For this review, take the finished solid that the model builds, in its own axes (mm). A direction names the side the tool comes from. Round coordinates to 2 decimals unless told otherwise and drop trailing zeros. Write each loop counter-clockwise with the first axis right and the second up, starting at its lowest first coordinate (ties: lowest second). Pieces come first, ordered by that corner, then holes.
from build123d import *

# Parameters (mm, degrees)
SKETCH1_R           = 11.7729
SKETCH1_R_2         = 1.016
BOSS_EXTRUDE1_DEPTH = 1.6256
SKETCH2_R           = 0.762
CUT_EXTRUDE1_DEPTH  = 17.728566112
SKETCH3_R           = 3.3655
SKETCH3_R_2         = 2.2606
BOSS_EXTRUDE2_DEPTH = 2.54
SKETCH4_R           = 2.6924
BOSS_EXTRUDE3_DEPTH = 0.8636
SKETCH5_R           = 2.2606
CUT_EXTRUDE2_DEPTH  = 1.27


with BuildPart() as part:
    # Sketch1 → Boss-Extrude1 (new body)
    with BuildSketch(Plane(origin=(0, 0, 0), x_dir=(1, 0, 0), z_dir=(0, 1, 0))):
        with Locations(Location((0, 0, 0), (0, 0, 270))):
            Circle(SKETCH1_R)
        with Locations(Location((0, 0, 0), (0, 0, 270))):
            Circle(SKETCH1_R_2, mode=Mode.SUBTRACT)
    extrude(amount=BOSS_EXTRUDE1_DEPTH)

    # Sketch2 → Cut-Extrude1 (cut, through all)
    with BuildSketch(Plane(origin=(0, 1.6256, 0), x_dir=(1, 0, 0), z_dir=(0, 1, 0))):
        with Locations(Location((8.0518, 0, 0), (0, 0, 270))):
            Circle(SKETCH2_R)
        with Locations(Location((-8.0518, 0, 0), (0, 0, 270))):
            Circle(SKETCH2_R)
    extrude(amount=-CUT_EXTRUDE1_DEPTH, mode=Mode.SUBTRACT)

    # Sketch3 → Boss-Extrude2 (add)
    with BuildSketch(Plane(origin=(0, 1.6256, 0), x_dir=(1, 0, 0), z_dir=(0, 1, 0))):
        with Locations(Location((0, 0, 0), (0, 0, 270))):
            Circle(SKETCH3_R)
        with Locations(Location((0, 0, 0), (0, 0, 270))):
            Circle(SKETCH3_R_2, mode=Mode.SUBTRACT)
    extrude(amount=BOSS_EXTRUDE2_DEPTH)

    # Sketch4 → Boss-Extrude3 (add)
    with BuildSketch(Plane.XZ):
        with Locations(Location((0, 0, 0), (0, 0, 90))):
            Circle(SKETCH4_R)
    extrude(amount=BOSS_EXTRUDE3_DEPTH)

    # Sketch5 → Cut-Extrude2 (cut)
    with BuildSketch(Plane.XZ.offset(0.8636)):
        with Locations(Location((0, 0, 0), (0, 0, 90))):
            Circle(SKETCH5_R)
    extrude(amount=-CUT_EXTRUDE2_DEPTH, mode=Mode.SUBTRACT)


solid = part.part
(1) We need section B-B, the plane x = 0. Give the boundary of the cut face in (y, z), and give its area (3 significant figures).
Geometry check:
outline: (-0.86, -2.69) - (0, -2.69) - (0, -11.77) - (1.63, -11.77) - (1.63, -3.37) - (4.17, -3.37) - (4.17, -2.26) - (1.63, -2.26) - (1.63, -1.02) - (0.41, -1.02) - (0.41, -2.26) - (-0.86, -2.26) - close; (-0.86, 2.26) - (0.41, 2.26) - (0.41, 1.02) - (1.63, 1.02) - (1.63, 2.26) - (4.17, 2.26) - (4.17, 3.37) - (1.63, 3.37) - (1.63, 11.77) - (0, 11.77) - (0, 2.69) - (-0.86, 2.69) - close
area: 40.3 mm2
(2) We need section D-D, the plane x = 4.25. Give the boundary of the cut face in (y, z).
Geometry check:
outline: (0, -10.98) - (1.63, -10.98) - (1.63, 10.98) - (0, 10.98) - close
(3) For pin 1 Ø2 at (x, y) = (-6, 0.5) entering from +Z; pin 2 Ø2 at (x, z) = (7.5, 6) entering from +Y; pin 3 Ø1 at (x, y) = (2, 1) entering from -Z; pin 4 Ø2.5 at (x, z) = (1, -1) entering from +Y, all flat-tipped, find the tip position at first contact; note any pin that passes through.
Geometry check:
pin 1: stops at z = 10.66
pin 2: stops at y = 1.63
pin 3: stops at z = -11.68
pin 4: stops at y = 4.17
(4) For line 1 along X through (y, z) = (1.1, 0); line 2 along Y through (x, z) = (2.75, -9); line 3 along Z through (x, y) = (0.5, 2.45), list the stretches that pass through material, from the lowest coordinate up.
Geometry check:
line 1: x = -11.77 to -8.81, -7.29 to -1.02, 1.02 to 7.29, 8.81 to 11.77
line 2: y = 0 to 1.63
line 3: z = -3.33 to -2.2, 2.2 to 3.33
(5) We need section A-A, the plane z = 0. State how many separate pieces and enclosed holes the cut face has, and give its area (3 significant figures).
Geometry check:
separate pieces: 4
enclosed holes: 0
area: 35.4 mm2
(6) Mouldability with a two-part tool opening along Z and no side actions: class faces 1 (the face through (2.838, 2.878, 1.809)), 2 (the face through (-1, 0.406, 1)), 3 (the face through (-8.344, 0.824, 0.704)), 4 (the face through (3, 0, 0)) as pulls with the +Z half, pulls with the -Z half, needs draft (parallel to the pull), parting line crosses it, or undercut.
Geometry check:
face 1: parting line crosses it
face 2: undercut
face 3: undercut
face 4: needs draft
(7) For faces 5 (the face through (1, 1.626, 1)), 6 (the face through (7.31, 0.82, -0.17)), 7 (the face through (-0.679, -0.237, 2.156)), list the 3-axis set-ups (+Z, -Z, +X, -X, +Y, -Y) from which the entire face can be reached by the end or side of a thin tool; tool diameter is ignored.
Geometry check:
face 5: +Y
face 6: +Y, -Y
face 7: -Y
(8) We need section C-C, the plane y = 3.8. Give the boundary of the cut face in (x, z), and give its area (3 significant figures).
Geometry check:
outline: circle Ø6.73 at (0, 0); hole circle Ø4.52 at (0, 0)
area: 19.5 mm2
